Check sheet for the modelled part. Datum: model origin and axes. Units: mm. Give positions to 0.01 mm unless a question says otherwise; leave off trailing zeros. Loops run counter-clockwise (first coordinate to the right, second up) from the corner with the lowest first, then second, coordinate; pieces in that order, holes last. Notation, with made-up numbers: (57.25, 89.5) - (69.25, 89.5) arc R32 ccw to (69.25, 125.5) - close; hole circle Ø5 at (-29.75, -12). An arc over 180 degrees is marked (long way). Answer in a Markdown table with one row per item. Add a question column.
(1) Go/stop test with a flat-tipped pin: P1, Ø4, axis at x = 13.26, z = 297, coming from the -Y side. Record where the tip stops, or that it passes through.
(2) Sectioned sample at B-B on z = 273. Enter the section's corners in (x, y) (3 decimals).
(3) Thickness scan on L1, parallel to Y at x = 13.25, z = 368; L2, parallel to X at y = 21.25, z = 261.5; L3, parallel to Z at x = 1.75, y = 12.7. Record the ranges inside material, lowest first.
(4) Sectioned sample at A-A on z = 500.3. Enter the section's corners in (x, y) (3 decimals), then the cut area to 3 significant figures.
Autodesk Inventor part; units mm, degrees
ref_plane "YZ Plane" through (0, 0, 0) normal (1, 0, 0) x (0, 1, 0)
ref_plane "XZ Plane" through (0, 0, 0) normal (0, 1, 0) x (-1, 0, 0)
ref_plane "XY Plane" through (0, 0, 0) normal (0, 0, 1) x (1, 0, 0)
sketch "Sketch1" plane through (0, 0, 0) normal (0, 0, 1) x (1, 0, 0)
  line L0 (3.7363, 0) -> (22.7863, 0)
  line L1 (25.9613, 3.175) -> (25.9613, 22.225)
  line L2 (22.7863, 25.4) -> (3.7363, 25.4)
  line L3 (0.5613, 22.225) -> (0.5613, 3.175)
  arc A0 (3.7363, 25.4) -> (0.5613, 22.225) centre (3.7363, 22.225) ccw
  arc A1 (0.5613, 3.175) -> (3.7363, 0) centre (3.7363, 3.175) ccw
  arc A2 (22.7863, 0) -> (25.9613, 3.175) centre (22.7863, 3.175) ccw
  arc A3 (25.9613, 22.225) -> (22.7863, 25.4) centre (22.7863, 22.225) ccw
  line L4 (3.7363, 23.749) -> (22.7863, 23.749)
  arc A4 (24.3103, 22.225) -> (22.7863, 23.749) centre (22.7863, 22.225) ccw
  line L5 (24.3103, 22.225) -> (24.3103, 3.175)
  arc A5 (22.7863, 1.651) -> (24.3103, 3.175) centre (22.7863, 3.175) ccw
  line L6 (22.7863, 1.651) -> (3.7363, 1.651)
  arc A6 (2.2123, 3.175) -> (3.7363, 1.651) centre (3.7363, 3.175) ccw
  line L7 (2.2123, 3.175) -> (2.2123, 22.225)
  arc A7 (3.7363, 23.749) -> (2.2123, 22.225) centre (3.7363, 22.225) ccw
  point P0 (0, 0)
  point P1 (0.5613, 0)
  point P2 (25.9613, 0)
  point P3 (0.5613, 25.4)
  dimension "d0" = 25.4
  dimension "d2" = 25.4
  dimension "d3" = 3.175
  dimension "d4" = 1.651
extrude "tube" add sketch "Sketch1" along normal blind 520.3
sketch "Sketch11" plane through (3.7363, 25.4, 0) normal (0, 1, 0) x (1, 0, 0)
  line L0 (19.05, 0) -> (0, 0)
  circle A0 centre (9.525, -20) radius 2.8743
  point P0 (-3.7363, 0)
  dimension "d83" = 20
hole "centerHole_cutOff" at (13.2613, 25.4, 20) direction (0, -1, 0) diameter 6.35 end through all
sketch "Sketch12" plane through (3.7363, 25.4, 0) normal (0, 1, 0) x (1, 0, 0)
  circle A0 centre (9.525, -20) radius 3.175
  circle A1 centre (9.525, -77) radius 2.5235
  point P0 (-3.7363, 0)
  dimension "d91" = 57
hole "collarHole" at (13.2613, 25.4, 77) direction (0, -1, 0) diameter 6.6 end through all
sketch "Sketch8" plane through (3.7363, 25.4, 520.3) normal (0, 1, 0) x (1, 0, 0)
  line L0 (0, 520.3) -> (0, 0)
  circle A0 centre (9.525, 73.3) radius 1.5875
  circle A1 centre (9.525, 223.3) radius 1.5875
  circle A2 centre (9.525, 373.3) radius 1.5875
  circle A3 centre (9.525, 500.3) radius 3.175
  point P0 (0, 518.1689)
  point P1 (-3.7363, 520.3)
  dimension "d43" = 3.175
  dimension "d47" = 150
  dimension "d99" = 127
hole "armAttach" at (13.2613, 25.4, 447) at (13.2613, 25.4, 297) at (13.2613, 25.4, 147) direction (0, -1, 0) diameter 4.5 end through all
sketch "Sketch6" plane through (25.9613, 3.175, 520.3) normal (1, 0, 0) x (0, 0, -1)
  line L0 (0, 0) -> (0, 19.05)
  circle A0 centre (20, 9.525) radius 2.9685
  point P0 (520.3, -3.175)
  dimension "d27" = 20
hole "ropeAttach" at (25.9613, 12.7, 500.3) direction (-1, 0, 0) diameter 8 end through all
sketch "Sketch13" plane through (3.7363, 25.4, 0) normal (0, 1, 0) x (1, 0, 0)
  circle A0 centre (9.525, -20) radius 3.175
  line L0 (9.525, -20) -> (9.525, -34.6812) construction
  line L1 (-12.9518, -21.6531) -> (31.0422, -47.0531)
  line L2 (0, -34.6812) -> (50.8, -34.6812) construction
  line L3 (-12.9518, 4.6365) -> (31.0422, 4.6365)
  line L4 (31.0422, -47.0531) -> (31.0422, 4.6365)
  line L5 (-12.9518, 4.6365) -> (-12.9518, -21.6531)
  point P0 (-3.7363, 0)
  dimension "d100" = 14.6812
  dimension "d101" = 50.8
  dimension "d102" = 30
extrude "angledEnd" cut sketch "Sketch13" against normal blind 50.8
equation "\"tube\" = 25.4"
properties part number "2f2ax1" material "Steel"
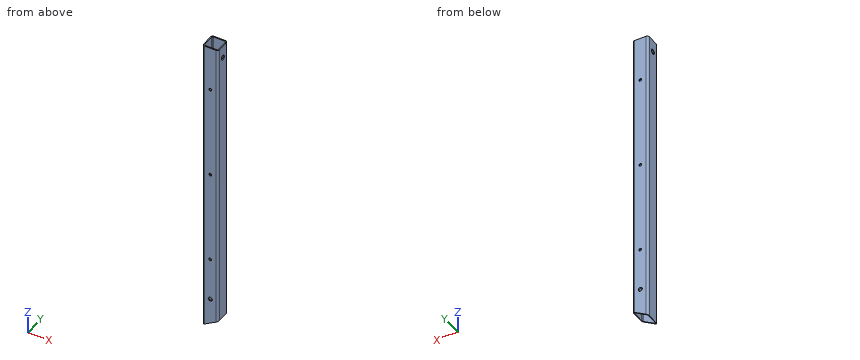
Reply:
| question | item | result |
|---|---|---|
| 1 | P1 | through |
| 2 | outline | (0.561, 3.175) arc R3.175 ccw to (3.736, 0) - (22.786, 0) arc R3.175 ccw to (25.961, 3.175) - (25.961, 22.225) arc R3.175 ccw to (22.786, 25.4) - (3.736, 25.4) arc R3.175 ccw to (0.561, 22.225) - close; hole (2.212, 3.175) arc R1.524 ccw to (3.736, 1.651) - (22.786, 1.651) arc R1.524 ccw to (24.31, 3.175) - (24.31, 22.225) arc R1.524 ccw to (22.786, 23.749) - (3.736, 23.749) arc R1.524 ccw to (2.212, 22.225) - close |
| 3 | L1 | 0 to 1.65, 23.75 to 25.4 |
| 3 | L2 | 0.56 to 2.21, 24.31 to 25.96 |
| 3 | L3 | 27.98 to 496.3, 504.3 to 520.3 |
| 4 | outline | (0.561, 3.175) arc R3.175 ccw to (3.736, 0) - (22.786, 0) arc R3.175 ccw to (25.961, 3.175) - (25.961, 8.7) - (24.31, 8.7) - (24.31, 3.175) arc R1.524 cw to (22.786, 1.651) - (3.736, 1.651) arc R1.524 cw to (2.212, 3.175) - (2.212, 8.7) - (0.561, 8.7) - close; (0.561, 16.7) - (2.212, 16.7) - (2.212, 22.225) arc R1.524 cw to (3.736, 23.749) - (22.786, 23.749) arc R1.524 cw to (24.31, 22.225) - (24.31, 16.7) - (25.961, 16.7) - (25.961, 22.225) arc R3.175 ccw to (22.786, 25.4) - (3.736, 25.4) arc R3.175 ccw to (0.561, 22.225) - close |
| 4 | area | 124 mm^2 |
